from build123d import *

# Parameters (mm, degrees)
SKETCH2_W           = 200
SKETCH2_H           = 100
BOSS_EXTRUDE1_DEPTH = 10.357742679
SKETCH4_W           = 10
SKETCH4_H           = 25
BOSS_EXTRUDE2_DEPTH = 150
SKETCH7_W           = 10
SKETCH7_H           = 25
BOSS_EXTRUDE3_DEPTH = 100


with BuildPart() as part:
    # Sketch2 → Boss-Extrude1 (new body)
    with BuildSketch(Plane(origin=(0, 0, 0), x_dir=(1, 0, 0), z_dir=(0, 1, 0))):
        Rectangle(SKETCH2_W, SKETCH2_H)
    extrude(amount=BOSS_EXTRUDE1_DEPTH)

    # Sketch4 → Boss-Extrude2 (add)
    with BuildSketch(Plane(origin=(0, 10.357742679, 0), x_dir=(1, 0, 0), z_dir=(0, 1, 0))):
        with Locations((-80, 0)):
            Rectangle(SKETCH4_W, SKETCH4_H)
        with Locations((-55, 0)):
            Rectangle(SKETCH4_W, SKETCH4_H)
    extrude(amount=BOSS_EXTRUDE2_DEPTH)

    # Sketch7 → Boss-Extrude3 (add)
    with BuildSketch(Plane(origin=(0, 10.357742679, 0), x_dir=(1, 0, 0), z_dir=(0, 1, 0))):
        with Locations((80, 0)):
            Rectangle(SKETCH7_W, SKETCH7_H)
        with Locations((55, 0)):
            Rectangle(SKETCH7_W, SKETCH7_H)
    extrude(amount=BOSS_EXTRUDE3_DEPTH)


solid = part.part
For this review, take the finished solid that the model builds, in its own axes (mm). A direction names the side the tool comes from. Give positions to 0.01 mm unless a question says otherwise; leave off trailing zeros. Order: outer loops, then holes, each group sorted by start corner. A loop starts at its lowest first (then second) coordinate and runs counter-clockwise, first axis right, second up. Notation, with made-up numbers: M 60.25,-30.75 L 99.25,-30.75 A11 ccw 99.25,-23.75 Z; hole C 0.25,34 d9. An arc over 180 degrees is marked long. Answer in a Markdown table with one row per item. Add a question column.
(1) Wall thickness on probe 1 along X at (y, z) = (61.5, -10); probe 2 along Y at (x, z) = (10, -23.5): over which ranges is each line inside the solid? List them lowest first. Write a range as [from, to].
(2) Consider section B-B on y = 146. State the section outline as (x, z) points, and give its area (3 significant figures).
(3) Consider section C-C on z = 8. State the section outline as (x, y) points.
(4) For pin 1 (11 mm diameter, centred on x = -57.5, y = 50, fed in from -Z); pin 2 (5 mm diameter, centred on x = 60.5, z = -14, fed in from +Y); pin 3 (10 mm diameter, centred on x = -53.5, z = -38.5, fed in from +Y), all flat-tipped, find the tip position at first contact; note any pin that passes through.
(5) Mouldability with a two-part tool opening along X and no side actions: class faces 4 (the face through (100, 5, 1)), 5 (the face through (-60, 84, 0)), 6 (the face through (-100, 5, 1)) as +X half, -X half, draft (parallel to the pull), parting line (faces both ways), or undercut.
(6) Consider section D-D on x = 82. State the section outline as (y, z) points.
(7) For faces 1 (the face through (-75, 84, 0)), 2 (the face through (55, 60, 12.5)), 3 (the face through (55, 110.358, 0)), list the 3-axis set-ups (+Z, -Z, +X, -X, +Y, -Y) from which the entire face can be reached by the end or side of a thin tool; tool diameter is ignored.
(8) Consider section A-A on y = 23.5. State the section outline as (x, z) points, and give its area (3 significant figures).
Evaluation:
| question | item | result |
|---|---|---|
| 1 | probe 1 | x = [-85, -75], [-60, -50], [50, 60], [75, 85] |
| 1 | probe 2 | y = [0, 10.36] |
| 2 | outline | M -85,-12.5 L -75,-12.5 L -75,12.5 L -85,12.5 Z; M -60,-12.5 L -50,-12.5 L -50,12.5 L -60,12.5 Z |
| 2 | area | 500 mm^2 |
| 3 | outline | M -100,0 L 100,0 L 100,10.36 L 85,10.36 L 85,110.36 L 75,110.36 L 75,10.36 L 60,10.36 L 60,110.36 L 50,110.36 L 50,10.36 L -50,10.36 L -50,160.36 L -60,160.36 L -60,10.36 L -75,10.36 L -75,160.36 L -85,160.36 L -85,10.36 L -100,10.36 Z |
| 4 | pin 1 | stops at z = -12.5 |
| 4 | pin 2 | stops at y = 110.36 |
| 4 | pin 3 | stops at y = 10.36 |
| 5 | face 4 | +X half |
| 5 | face 5 | undercut |
| 5 | face 6 | -X half |
| 6 | outline | M 0,-50 L 10.36,-50 L 10.36,-12.5 L 110.36,-12.5 L 110.36,12.5 L 10.36,12.5 L 10.36,50 L 0,50 Z |
| 7 | face 1 | +Z, -Z, +Y |
| 7 | face 2 | +Z, +X, -X, +Y |
| 7 | face 3 | +Z, -Z, +X, +Y |
| 8 | outline | M -85,-12.5 L -75,-12.5 L -75,12.5 L -85,12.5 Z; M -60,-12.5 L -50,-12.5 L -50,12.5 L -60,12.5 Z; M 50,-12.5 L 60,-12.5 L 60,12.5 L 50,12.5 Z; M 75,-12.5 L 85,-12.5 L 85,12.5 L 75,12.5 Z |
| 8 | area | 1,000 mm^2 |
